```python
from build123d import *

# Parameters (mm, degrees)
SKETCH_1_R      = 3.5
SKETCH_1_R_2    = 2
EXTRUDE_2_DEPTH = 3


with BuildPart() as part:
    # ｽｹｯﾁ1 → ﾎﾞｽ - 押し出し2 (new body)
    # profile 1 of 4: a face of its own
    with BuildSketch(Plane(origin=(0, 0, 0), x_dir=(1, 0, 0), z_dir=(0, 1, 0))):
        with BuildLine():
            Line((-30.418207164, -18.784024388), (-6.418207164, -18.784024388))
            ThreePointArc((-6.418207164, -18.784024388), (-9.918207164, -15.284024388), (-6.418207164, -11.784024388))
            Line((-6.418207164, -11.784024388), (-30.418207164, -11.784024388))
            ThreePointArc((-30.418207164, -11.784024388), (-27.94333343, -12.809150654), (-26.918207164, -15.284024388))
            ThreePointArc((-26.918207164, -15.284024388), (-27.94333343, -17.758898122), (-30.418207164, -18.784024388))
        make_face()
    # profile 2 of 4: a face of its own
    with BuildSketch(Plane(origin=(0, 0, 0), x_dir=(1, 0, 0), z_dir=(0, 1, 0))):
        with Locations((-30.418207164, -15.284024388)):
            Circle(SKETCH_1_R)
        with Locations(Location((-30.418207164, -15.284024388, 0), (0, 0, 270))):
            Circle(SKETCH_1_R_2, mode=Mode.SUBTRACT)
    # profile 3 of 4: a face of its own
    with BuildSketch(Plane(origin=(0, 0, 0), x_dir=(1, 0, 0), z_dir=(0, 1, 0))):
        with Locations((-6.418207164, -15.284024388)):
            Circle(SKETCH_1_R)
        with Locations(Location((-6.418207164, -15.284024388, 0), (0, 0, 270))):
            Circle(SKETCH_1_R_2, mode=Mode.SUBTRACT)
    # profile 4 of 4: a face of its own
    with BuildSketch(Plane(origin=(0, 0, 0), x_dir=(1, 0, 0), z_dir=(0, 1, 0))):
        with BuildLine():
            ThreePointArc((-2.918207164, -15.284024388), (-3.260445919, -16.793509042), (-4.220232261, -18.007791325))
            Line((-4.220232261, -18.007791325), (28.091680373, -4.237751216))
            Line((28.091680373, -4.237751216), (32.606722729, -8.053690239))
            Line((32.606722729, -8.053690239), (35.636170503, -6.538966352))
            Line((35.636170503, -6.538966352), (30.97548162, 0.772489334))
            Line((30.97548162, 0.772489334), (-6.418207164, -11.784024388))
            ThreePointArc((-6.418207164, -11.784024388), (-3.94333343, -12.809150654), (-2.918207164, -15.284024388))
        make_face()
    extrude(amount=EXTRUDE_2_DEPTH)


solid = part.part
```
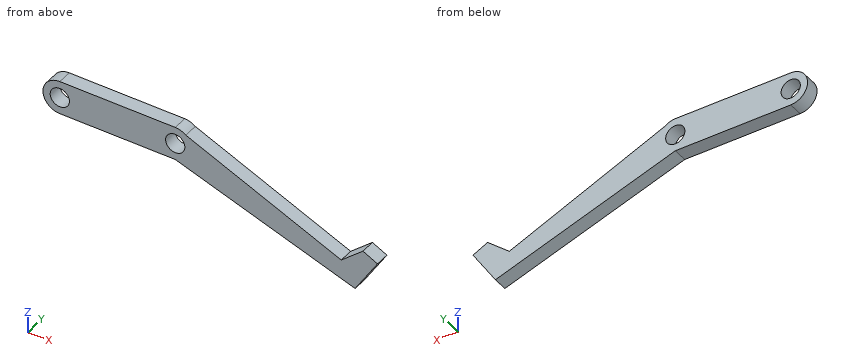
Read the model definition and answer for the solid it produces. Units are mm, in the model's axes. Coordinates: 2 decimals unless noted, no trailing zeros. Loops run counter-clockwise (first coordinate to the right, second up) from the corner with the lowest first, then second, coordinate; pieces in that order, holes last.
(1) The part is cut by section C-C (x = 8.5). Determine the outline of the cut face in (y, z), and give its area (3 significant figures).
Solution:
outline: (0, 6.77) - (3, 6.77) - (3, 12.59) - (0, 12.59) - close
area: 17.4 mm2
(2) The part is cut by section A-A (y = 1.45). Determine the outline of the cut face in (x, z).
Solution:
outline: (-30.42, 11.78) - (-6.42, 11.78) - (30.98, -0.77) - (35.64, 6.54) - (32.61, 8.05) - (28.09, 4.24) - (-4.22, 18.01) arc R3.5 ccw to (-6.42, 18.78) - (-30.42, 18.78) arc R3.5 ccw to start; hole circle Ø4 at (-30.42, 15.28); hole circle Ø4 at (-6.42, 15.28)
(3) The part is cut by section B-B (z = 5.25). Determine the outline of the cut face in (x, y), and give its area (3 significant figures).
Solution:
outline: (13.04, 0) - (25.72, 0) - (25.72, 3) - (13.04, 3) - close; (29.29, 0) - (34.81, 0) - (34.81, 3) - (29.29, 3) - close
area: 54.6 mm2
(4) The part is cut by section D-D (x = -18.5). Determine the outline of the cut face in (y, z), and give its area (3 significant figures).
Solution:
outline: (0, 11.78) - (3, 11.78) - (3, 18.78) - (0, 18.78) - close
area: 21.0 mm2
(5) A flat-ended cylindrical pin translates along its axis: pin 1 Ø1 at (x, z) = (9, 14.5) entering from -Y. Find the tip coordinate at first contact, or state that the pin passes through.
Solution:
pin 1: passes through
(6) Consider line 1 along X through (y, z) = (1.7, 13.5); line 2 along Z through (x, y) = (-17.5, 2.25); line 3 along Z through (x, y) = (-29, 1.5). Determine where each line is inside the solid, lowest interval first.
Solution:
line 1: x = -33.43 to -31.32, -29.51 to -7.32, -5.51 to 6.36
line 2: z = 11.78 to 18.78
line 3: z = 11.78 to 13.87, 16.69 to 18.78
